For this review, take the finished solid that the model builds, in its own axes (mm). A direction names the side the tool comes from. Coordinates: 2 decimals unless noted, no trailing zeros. Loops run counter-clockwise (first coordinate to the right, second up) from the corner with the lowest first, then second, coordinate; pieces in that order, holes last. Notation, with made-up numbers: M 89.5,46.5 L 136.5,46.5 A20 cw 136.5,61.5 Z; hole C 39,-8.75 d8. An arc over 180 degrees is marked long. Answer as a JSON object with one key per item and string values. Group by question number.
Item 1: Add section B-B (y = 3.25). Count the separate pieces of the cut face and the enclosed holes in it, then the cut area to 3 significant figures.
Item 2: Add section A-A (x = -15). State the section outline as (y, z) points.
Item 3: Tool access review of faces 1 (the face through (-1.94, 5.01, -6.73)), 2 (the face through (-30, 3, -2)), 3 (the face through (-17.67, 6.26, -3.27)): name each direction out of +Z, -Z, +X, -X, +Y, -Y from which nothing blocks a thin tool from reaching the whole face with its end or side.
Item 4: Add section D-D (z = -21.5). State the section outline as (x, y) points.
Item 5: Insertion check: pin 1 (1.5 mm diameter, centred on x = -19, y = 2, fed in from -Z). The pin has a flat end and moves straight along its axis. Give the tip position at first contact, or say it passes through.
Item 6: Mouldability with a two-part tool opening along Y and no side actions: class faces 4 (the face through (-1.71, 1.49, -15.02)), 5 (the face through (-4.886, 6.259, -4.239)), 6 (the face through (-3.237, 3.204, -16.987)) as +Y half, -Y half, draft (parallel to the pull), parting line (faces both ways), or undercut.
Item 7: Wall thickness on L1, parallel to Z at x = -1.75, y = 4.25; L2, parallel to Y at x = -15, z = -1.95; L3, parallel to X at y = 2, z = -2.5: over which ranges is each line inside the solid? List them lowest first. Write a range as from..to.
Item 8: Add section C-C (z = -1.5). State the section outline as (x, y) points, then the cut area to 3 significant figures.
Autodesk Inventor part; units mm, degrees
ref_plane "YZ Plane" through (0, 0, 0) normal (1, 0, 0) x (0, 1, 0)
ref_plane "XZ Plane" through (0, 0, 0) normal (0, 1, 0) x (-1, 0, 0)
ref_plane "XY Plane" through (0, 0, 0) normal (0, 0, 1) x (1, 0, 0)
sketch "Szkic1" plane through (0, 0, 0) normal (0, 1, 0) x (-1, 0, 0)
  line L0 (0, 0) -> (30, 0)
  line L1 (30, 0) -> (30, -3.5)
  line L2 (30, -3.5) -> (4, -3.5)
  line L3 (4, -3.5) -> (2.5, -30)
  line L4 (2.5, -30) -> (0, -30)
  line L5 (0, -30) -> (0, 0)
  dimension "d0" = 30
  dimension "d1" = 30
  dimension "d2" = 3.5
  dimension "d3" = 2.5
  dimension "d4" = 4
extrude "Wyciągnięcie proste1" add sketch "Szkic1" along normal blind 6.5
sketch "Szkic2" plane through (0, 0, 0) normal (1, 0, 0) x (0, 0, -1)
  line L0 (0, 0) -> (30, 0)
  line L1 (30, 0) -> (30, 6.5)
  line L2 (0, 6.5) -> (30, 6.5)
  line L3 (0, 0) -> (0, 6.5)
  line L4 (30, 3.25) -> (0, 3.25) construction
  line L5 (18.25, 5.25) -> (27, 5.25)
  line L6 (27, 5.25) -> (27, 1.25)
  line L7 (27, 1.25) -> (18.25, 1.25)
  line L8 (18.25, 1.25) -> (18.25, 5.25)
  line L9 (18.25, 5.25) -> (27, 1.25) construction
  line L10 (27, 5.25) -> (18.25, 1.25) construction
  line L11 (6.5, 5.25) -> (15.25, 5.25)
  line L12 (15.25, 5.25) -> (15.25, 1.25)
  line L13 (15.25, 1.25) -> (6.5, 1.25)
  line L14 (6.5, 1.25) -> (6.5, 5.25)
  line L15 (6.5, 5.25) -> (15.25, 1.25) construction
  line L16 (15.25, 5.25) -> (6.5, 1.25) construction
  line L17 (3.5, 0) -> (3.5, 6.5)
  point P0 (22.625, 3.25)
  point P1 (10.875, 3.25)
  dimension "d7" = 26.5
  dimension "d8" = 3
  dimension "d9" = 3
  dimension "d10" = 3
  dimension "d11" = 4
extrude "Wyciągnięcie proste2" cut sketch "Szkic2" against normal up to surface contours L5 L6 L7 L8 | L11 L12 L13 L14 surface through (-2.5, 0, -30) normal (-0.9984018, 0, -0.0565133)
sketch "Szkic3" plane through (-30, 0, 0) normal (0, 0, 1) x (1, 0, 0)
  line L0 (0, 0) -> (30, 0)
  line L1 (30, 0) -> (30, 6.5)
  line L2 (0, 6.5) -> (30, 6.5) construction
  line L3 (0, 0) -> (0, 6.5)
  line L4 (0, 3.25) -> (30, 3.25) construction
  circle A0 centre (15, 3.25) radius 1.75
  circle A1 centre (5, 3.25) radius 1.75
  dimension "d14" = 3.5
  dimension "d15" = 15
  dimension "d16" = 10
extrude "Wyciągnięcie proste3" cut sketch "Szkic3" against normal up to surface (3.5 mm away)
chamfer "Faza1" distance 2 angle 45 1 edges at (-4, 3.25, -3.5)
fillet "Zaokrąglenie1" radius 0.8 16 edges at (-1.25, 6.5, -30) (-1.25, 0, -30) (-15, 6.5, 0) (-15, 0, 0) (-18, 0, -3.5) (-18, 6.5, -3.5) (-4.9435, 6.5, -4.4984) (-4.9435, 0, -4.4984) (-1.9151, 1.25, -6.5) (-1.9151, 5.25, -6.5) (-1.6675, 5.25, -15.25) (-1.6675, 1.25, -15.25) (-1.5825, 1.25, -18.25) (-1.5825, 5.25, -18.25) (-1.3349, 5.25, -27) (-1.3349, 1.25, -27)
fillet "Zaokrąglenie2" radius 0.4 4 edges at (-16.75, 3.25, -3.5) (-16.75, 3.25, 0) (-26.75, 3.25, 0) (-26.75, 3.25, -3.5)
equation "\"d9\" = d8"
properties part number "noga2"
From the geometry:
{
 "1": {"separate pieces": "5", "enclosed holes": "0", "area": "111 mm²"},
 "2": {"outline": "M 0,-2.7 A0.8 ccw 0.8,-3.5 L 1.1,-3.5 A0.4 ccw 1.5,-3.1 L 1.5,-0.4 A0.4 ccw 1.1,0 L 0.8,0 A0.8 ccw 0,-0.8 Z; M 5,-3.1 A0.4 ccw 5.4,-3.5 L 5.7,-3.5 A0.8 ccw 6.5,-2.7 L 6.5,-0.8 A0.8 ccw 5.7,0 L 5.4,0 A0.4 ccw 5,-0.4 Z"},
 "3": {"face 1": "+X, -X", "face 2": "+Z, -Z, -X, +Y, -Y", "face 3": "-Z, -X, +Y"},
 "4": {"outline": "M -2.98,0 L 0,0 L 0,1.25 L -2.98,1.25 Z; M -2.98,5.25 L 0,5.25 L 0,6.5 L -2.98,6.5 Z"},
 "5": {"pin 1": "stops at z = -3.5"},
 "6": {"face 4": "undercut", "face 5": "+Y half", "face 6": "draft"},
 "7": {"L1": "z = -30..-27, -18.25..-15.25, -6.5..0", "L2": "y = 0..1.5, 5..6.5", "L3": "x = -30..-26.22, -23.78..-16.22, -13.78..0"},
 "8": {"outline": "M -30,0 L 0,0 L 0,6.5 L -30,6.5 Z; hole C -25,3.25 d3.5; hole C -15,3.25 d3.5", "area": "176 mm²"}
}
